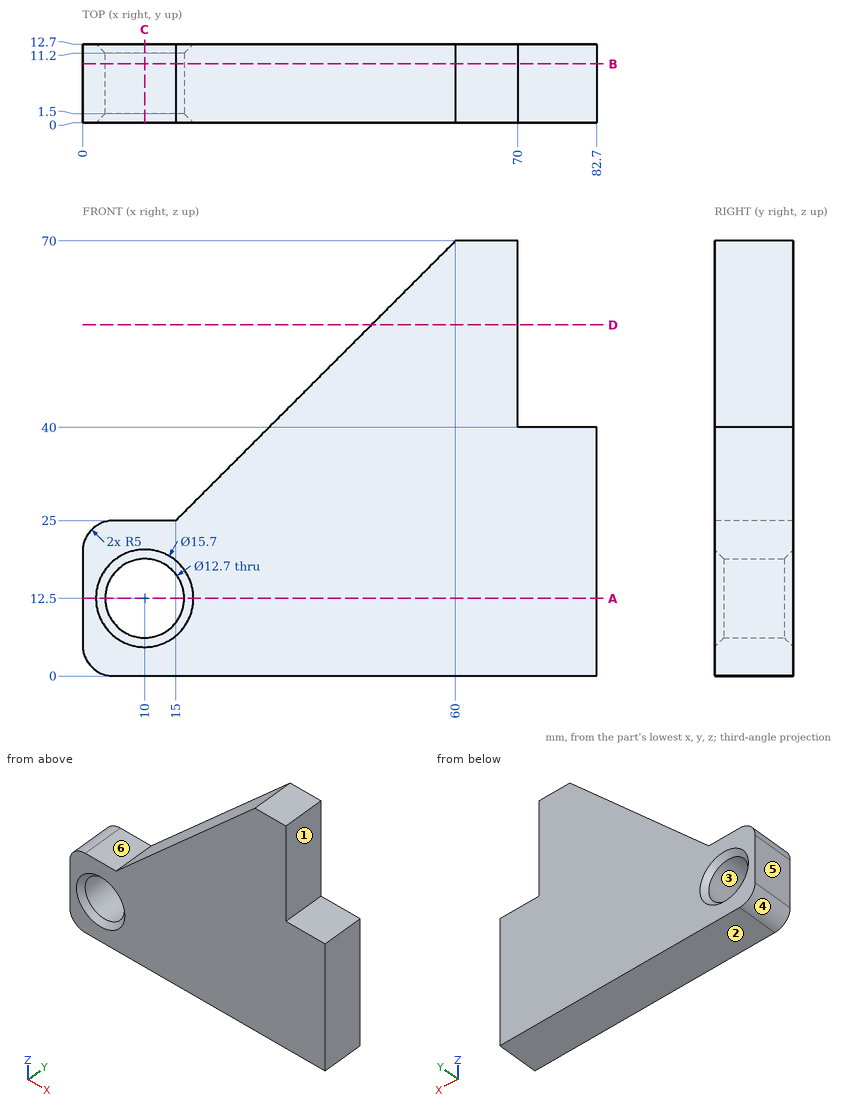
Drawing for the job (mm, zero at the part's lowest x, y, z). A direction names the side the tool comes from. Round coordinates to 2 decimals unless told otherwise and drop trailing zeros. Write each loop counter-clockwise with the first axis right and the second up, starting at its lowest first coordinate (ties: lowest second). Pieces come first, ordered by that corner, then holes. Notation, with made-up numbers: (-20, 67.5) - (-4, 67.5) arc R6 cw to (-4, 77.5) - close; hole circle Ø8 at (73.25, -11). An arc over 180 degrees is marked (long way). Return JSON: item names as keys, results as strings. Group by question number.
Item 1: 3-axis set-ups, long thin cutter, end or side, ignore diameter. For the marked faces 1 and 2: which of +Z, -Z, +X, -X, +Y, -Y reach the whole face in a straight line?
Item 2: Band-saw the part on A-A on z = 12.5. List the corners of the cut face in (x, y).
Item 3: Band-saw the part on B-B on y = 9.5. List the corners of the cut face in (x, z), plus the area to 3 significant figures.
Item 4: Mould opens along Z. For the marked faces 3, 4, 5 and 6 say: +Z half, -Z half, draft (parallel to the pull), parting line (faces both ways), or undercut.
Item 5: Band-saw the part on C-C on x = 10. List the corners of the cut face in (y, z), plus the area to 3 significant figures.
Item 6: Band-saw the part on D-D on z = 56.5. List the corners of the cut face in (x, y).
Item 7: Flat gauge pins, fed straight in: pin 1 Ø6.5 at (x, y) = (79, 8) entering from +Z; pin 2 Ø1.5 at (y, z) = (4, 48) entering from +X; pin 3 Ø14.5 at (x, z) = (10, 12.5) entering from -Y. Where does each tip first touch, or does it go through?
Item 8: Probe probe 1 along Z at (x, y) = (10, 8.5); probe 2 along X at (y, z) = (1, 18.5); probe 3 along X at (y, z) = (2, 8). List the from-to ranges inside material, lowest first.
Resolved:
{
 "1": {"face 1": "+Z, +X, +Y, -Y", "face 2": "-Z, +X, -X, +Y, -Y"},
 "2": {"outline": "(0, 0) - (2.15, 0) - (3.65, 1.5) - (3.65, 11.2) - (2.15, 12.7) - (0, 12.7) - close; (16.35, 1.5) - (17.85, 0) - (82.7, 0) - (82.7, 12.7) - (17.85, 12.7) - (16.35, 11.2) - close"},
 "3": {"outline": "(0, 5) arc R5 ccw to (5, 0) - (82.7, 0) - (82.7, 40) - (70, 40) - (70, 70) - (60, 70) - (15, 25) - (5, 25) arc R5 ccw to (0, 20) - close; hole circle Ø12.7 at (10, 12.5)", "area": "3,580 mm²"},
 "4": {"face 3": "undercut", "face 4": "-Z half", "face 5": "draft", "face 6": "+Z half"},
 "5": {"outline": "(0, 0) - (12.7, 0) - (12.7, 4.65) - (11.2, 6.15) - (1.5, 6.15) - (0, 4.65) - close; (0, 20.35) - (1.5, 18.85) - (11.2, 18.85) - (12.7, 20.35) - (12.7, 25) - (0, 25) - close", "area": "152 mm²"},
 "6": {"outline": "(46.5, 0) - (70, 0) - (70, 12.7) - (46.5, 12.7) - close"},
 "7": {"pin 1": "stops at z = 40", "pin 2": "stops at x = 70", "pin 3": "stops at y = 0.6"},
 "8": {"probe 1": "z = 0 to 6.15, 18.85 to 25", "probe 2": "x = 0 to 6.7, 13.3 to 82.7", "probe 3": "x = 0 to 5.52, 14.48 to 82.7"}
}
